Work out the finished part from the listing and answer in its coordinate system (mm). A direction names the side the tool comes from. Give positions to 0.01 mm unless a question says otherwise; leave off trailing zeros. Loops run counter-clockwise (first coordinate to the right, second up) from the corner with the lowest first, then second, coordinate; pieces in that order, holes last.
```python
from build123d import *

# Parameters (mm, degrees)
F1_DEPTH = 25.4
F2_R     = 9.525
F3_DEPTH = 25.4


with BuildPart() as f1:
    # F0 (on Front) → F1 (new body)
    with BuildSketch(Plane.XZ):
        with BuildLine():
            Line((-3.960718, 18.633712), (-3.432622, 16.149217))
            ThreePointArc((-3.432622, 16.149217), (-5.101871, 15.701943), (-6.715222, 15.082636))
            Line((-6.715222, 15.082636), (-7.748333, 17.403041))
            ThreePointArc((-7.748333, 17.403041), (-9.085269, 18.342204), (-10.660947, 18.774246))
            Line((-10.660947, 18.774246), (-10.795276, 18.697967))
            Line((-10.795276, 18.697967), (-10.9285, 18.619774))
            ThreePointArc((-10.9285, 18.619774), (-11.34218, 17.039175), (-11.197309, 15.411774))
            Line((-11.197309, 15.411774), (-9.704335, 13.356871))
            ThreePointArc((-9.704335, 13.356871), (-11.047346, 12.269321), (-12.269321, 11.047346))
            Line((-12.269321, 11.047346), (-14.156909, 12.746938))
            ThreePointArc((-14.156909, 12.746938), (-15.760252, 13.061125), (-17.375434, 12.814929))
            Line((-17.375434, 12.814929), (-17.467124, 12.690608))
            Line((-17.467124, 12.690608), (-17.557026, 12.564989))
            ThreePointArc((-17.557026, 12.564989), (-17.292054, 10.952781), (-16.497784, 9.525))
            Line((-16.497784, 9.525), (-14.298079, 8.255))
            ThreePointArc((-14.298079, 8.255), (-15.082636, 6.715222), (-15.701943, 5.101871))
            Line((-15.701943, 5.101871), (-18.117627, 5.886774))
            ThreePointArc((-18.117627, 5.886774), (-19.710145, 5.52166), (-21.08555, 4.639795))
            Line((-21.08555, 4.639795), (-21.118747, 4.488928))
            Line((-21.118747, 4.488928), (-21.149783, 4.337602))
            ThreePointArc((-21.149783, 4.337602), (-20.251975, 2.972551), (-18.945642, 1.991267))
            Line((-18.945642, 1.991267), (-16.419556, 1.725765))
            ThreePointArc((-16.419556, 1.725765), (-16.51, 0), (-16.419556, -1.725765))
            Line((-16.419556, -1.725765), (-18.945642, -1.991267))
            ThreePointArc((-18.945642, -1.991267), (-20.251975, -2.972551), (-21.149783, -4.337602))
            Line((-21.149783, -4.337602), (-21.118747, -4.488928))
            Line((-21.118747, -4.488928), (-21.08555, -4.639795))
            ThreePointArc((-21.08555, -4.639795), (-19.710145, -5.52166), (-18.117627, -5.886774))
            Line((-18.117627, -5.886774), (-15.701943, -5.101871))
            ThreePointArc((-15.701943, -5.101871), (-15.082636, -6.715222), (-14.298079, -8.255))
            Line((-14.298079, -8.255), (-16.497784, -9.525))
            ThreePointArc((-16.497784, -9.525), (-17.292054, -10.952781), (-17.557026, -12.564989))
            Line((-17.557026, -12.564989), (-17.467124, -12.690608))
            Line((-17.467124, -12.690608), (-17.375434, -12.814929))
            ThreePointArc((-17.375434, -12.814929), (-15.760252, -13.061125), (-14.156909, -12.746938))
            Line((-14.156909, -12.746938), (-12.269321, -11.047346))
            ThreePointArc((-12.269321, -11.047346), (-11.047346, -12.269321), (-9.704335, -13.356871))
            Line((-9.704335, -13.356871), (-11.197309, -15.411774))
            ThreePointArc((-11.197309, -15.411774), (-11.34218, -17.039175), (-10.9285, -18.619774))
            Line((-10.9285, -18.619774), (-10.795276, -18.697967))
            Line((-10.795276, -18.697967), (-10.660947, -18.774246))
            ThreePointArc((-10.660947, -18.774246), (-9.085269, -18.342204), (-7.748333, -17.403041))
            Line((-7.748333, -17.403041), (-6.715222, -15.082636))
            ThreePointArc((-6.715222, -15.082636), (-5.101871, -15.701943), (-3.432622, -16.149217))
            Line((-3.432622, -16.149217), (-3.960718, -18.633712))
            ThreePointArc((-3.960718, -18.633712), (-3.43114, -20.179342), (-2.410337, -21.455031))
            Line((-2.410337, -21.455031), (-2.256827, -21.472277))
            Line((-2.256827, -21.472277), (-2.103086, -21.487325))
            ThreePointArc((-2.103086, -21.487325), (-0.839359, -20.451749), (0, -19.05))
            Line((0, -19.05), (0, -16.51))
            ThreePointArc((0, -16.51), (1.725765, -16.419556), (3.432622, -16.149217))
            Line((3.432622, -16.149217), (3.960718, -18.633712))
            ThreePointArc((3.960718, -18.633712), (5.073175, -19.830316), (6.524595, -20.580519))
            Line((6.524595, -20.580519), (6.671848, -20.533836))
            Line((6.671848, -20.533836), (6.818418, -20.48505))
            ThreePointArc((6.818418, -20.48505), (7.551683, -19.025), (7.748333, -17.403041))
            Line((7.748333, -17.403041), (6.715222, -15.082636))
            ThreePointArc((6.715222, -15.082636), (8.255, -14.298079), (9.704335, -13.356871))
            Line((9.704335, -13.356871), (11.197309, -15.411774))
            ThreePointArc((11.197309, -15.411774), (12.700292, -16.052449), (14.331365, -16.147448))
            Line((14.331365, -16.147448), (14.4469, -16.044907))
            Line((14.4469, -16.044907), (14.560955, -15.940724))
            ThreePointArc((14.560955, -15.940724), (14.63697, -14.308657), (14.156909, -12.746938))
            Line((14.156909, -12.746938), (12.269321, -11.047346))
            ThreePointArc((12.269321, -11.047346), (13.356871, -9.704335), (14.298079, -8.255))
            Line((14.298079, -8.255), (16.497784, -9.525))
            ThreePointArc((16.497784, -9.525), (18.131414, -9.498968), (19.660112, -8.922336))
            Line((19.660112, -8.922336), (19.723951, -8.781669))
            Line((19.723951, -8.781669), (19.785771, -8.640102))
            ThreePointArc((19.785771, -8.640102), (19.191393, -7.118216), (18.117627, -5.886774))
            Line((18.117627, -5.886774), (15.701943, -5.101871))
            ThreePointArc((15.701943, -5.101871), (16.149217, -3.432622), (16.419556, -1.725765))
            Line((16.419556, -1.725765), (18.945642, -1.991267))
            ThreePointArc((18.945642, -1.991267), (20.427449, -1.303029), (21.589447, -0.154472))
            Line((21.589447, -0.154472), (21.590553, 0))
            Line((21.590553, 0), (21.589447, 0.154472))
            ThreePointArc((21.589447, 0.154472), (20.427449, 1.303029), (18.945642, 1.991267))
            Line((18.945642, 1.991267), (16.419556, 1.725765))
            ThreePointArc((16.419556, 1.725765), (16.149217, 3.432622), (15.701943, 5.101871))
            Line((15.701943, 5.101871), (18.117627, 5.886774))
            ThreePointArc((18.117627, 5.886774), (19.191393, 7.118216), (19.785771, 8.640102))
            Line((19.785771, 8.640102), (19.723951, 8.781669))
            Line((19.723951, 8.781669), (19.660112, 8.922336))
            ThreePointArc((19.660112, 8.922336), (18.131414, 9.498968), (16.497784, 9.525))
            Line((16.497784, 9.525), (14.298079, 8.255))
            ThreePointArc((14.298079, 8.255), (13.356871, 9.704335), (12.269321, 11.047346))
            Line((12.269321, 11.047346), (14.156909, 12.746938))
            ThreePointArc((14.156909, 12.746938), (14.63697, 14.308657), (14.560955, 15.940724))
            Line((14.560955, 15.940724), (14.4469, 16.044907))
            Line((14.4469, 16.044907), (14.331365, 16.147448))
            ThreePointArc((14.331365, 16.147448), (12.700292, 16.052449), (11.197309, 15.411774))
            Line((11.197309, 15.411774), (9.704335, 13.356871))
            ThreePointArc((9.704335, 13.356871), (8.255, 14.298079), (6.715222, 15.082636))
            Line((6.715222, 15.082636), (7.748333, 17.403041))
            ThreePointArc((7.748333, 17.403041), (7.551683, 19.025), (6.818418, 20.48505))
            Line((6.818418, 20.48505), (6.671848, 20.533836))
            Line((6.671848, 20.533836), (6.524595, 20.580519))
            ThreePointArc((6.524595, 20.580519), (5.073175, 19.830316), (3.960718, 18.633712))
            Line((3.960718, 18.633712), (3.432622, 16.149217))
            ThreePointArc((3.432622, 16.149217), (1.725765, 16.419556), (0, 16.51))
            Line((0, 16.51), (0, 19.05))
            ThreePointArc((0, 19.05), (-0.839359, 20.451749), (-2.103086, 21.487325))
            Line((-2.103086, 21.487325), (-2.256827, 21.472277))
            Line((-2.256827, 21.472277), (-2.410337, 21.455031))
            ThreePointArc((-2.410337, 21.455031), (-3.43114, 20.179342), (-3.960718, 18.633712))
        make_face()
    extrude(amount=F1_DEPTH)

    # F2 (on face) → F3 (cut)
    with BuildSketch(Plane.XZ.offset(25.4)):
        Circle(F2_R)
    extrude(amount=-F3_DEPTH, mode=Mode.SUBTRACT)


solid = f1.part
```
Q1. Section B-B on z = -7 is taken. Give the vertices of the cut face in (x, y), plus the area to 3 significant figures.
Q2. Given pin 1 (1 mm diameter, centred on y = -14, z = 13, fed in from -X); pin 2 (5 mm diameter, centred on x = -13.5, y = -21.5, fed in from +Z); pin 3 (0.8 mm diameter, centred on y = -13.5, z = 17.5, fed in from +X), each flat-ended and moving along its own axis, determine where each tip first touches the part or whether it passes through.
Q3. Determine the mould class of faces 5 (the face through (16.93, -12.52, -5.5)), 6 (the face through (-3.44, -12.52, -20.16)), 7 (the face through (17.7, -12.52, 1.86)), 8 (the face through (-13.2, -12.522, 11.885)) for opening direction Z: +Z half, -Z half, draft (parallel to the pull), parting line (faces both ways), or undercut.
Q4. Section C-C on x = 10.5 is taken. Give the vertices of the cut face in (y, z).
Q5. Section A-A on z = 18 is taken. Give the vertices of the cut face in (x, y).
Q6. Which of the six approach directions +Z, -Z, +X, -X, +Y, -Y give full straight-line access (tool end or side, diameter ignored) to faces 1 (the face through (-11.029, -12.522, 12.286)), 2 (the face through (19.203, -12.522, -7.138)), 3 (the face through (-10.44, -12.52, -14.37)), 4 (the face through (5.055, -12.522, -19.816))?
Q7. Consider line 1 along X through (y, z) = (-8.25, -14.5); line 2 along Z through (x, y) = (-2, -14.25); line 3 along X through (y, z) = (-20.5, 19.5). Determine where each line is inside the solid, lowest interval first.
Check result:
1. outline: (-14.95, -25.4) - (-6.46, -25.4) - (-6.46, 0) - (-14.95, 0) - close; (6.46, -25.4) - (19.12, -25.4) - (19.12, 0) - (6.46, 0) - close
1. area: 537 mm2
2. pin 1: stops at x = -17.56
2. pin 2: stops at z = 18.46
2. pin 3: stops at x = 7.75
3. face 5: undercut
3. face 6: -Z half
3. face 7: undercut
3. face 8: +Z half
4. outline: (-25.4, -14.45) - (0, -14.45) - (0, 14.45) - (-25.4, 14.45) - close
5. outline: (-11.16, -25.4) - (-8.48, -25.4) - (-8.48, 0) - (-11.16, 0) - close; (-3.83, -25.4) - (0, -25.4) - (0, 0) - (-3.83, 0) - close; (3.83, -25.4) - (7.74, -25.4) - (7.74, 0) - (3.83, 0) - close
6. face 1: +Y, -Y
6. face 2: +X, +Y, -Y
6. face 3: -X, +Y, -Y
6. face 4: -Z, +Y, -Y
7. line 1: x = -10.53 to 7.89, 10.53 to 14.66
7. line 2: z = -21.43 to -9.31, 9.31 to 21.43
7. line 3: x = -3.74 to -0.2, 4.68 to 7.38
